Print and shaded views of the part. All mm, measured from the part's lowest x, y and z. A direction names the side the tool comes from. Give positions to 0.01 mm unless a question says otherwise; leave off trailing zeros. Loops run counter-clockwise (first coordinate to the right, second up) from the corner with the lowest first, then second, coordinate; pieces in that order, holes last. Notation, with made-up numbers: (31, -12.75) -> (47, -12.75) arc R20 cw to (47, 13.25) -> close; hole circle Ø4 at (-38.5, -18.75). An arc over 180 degrees is marked (long way). Answer as a JSON object with one key per item and string values. Group by question number.
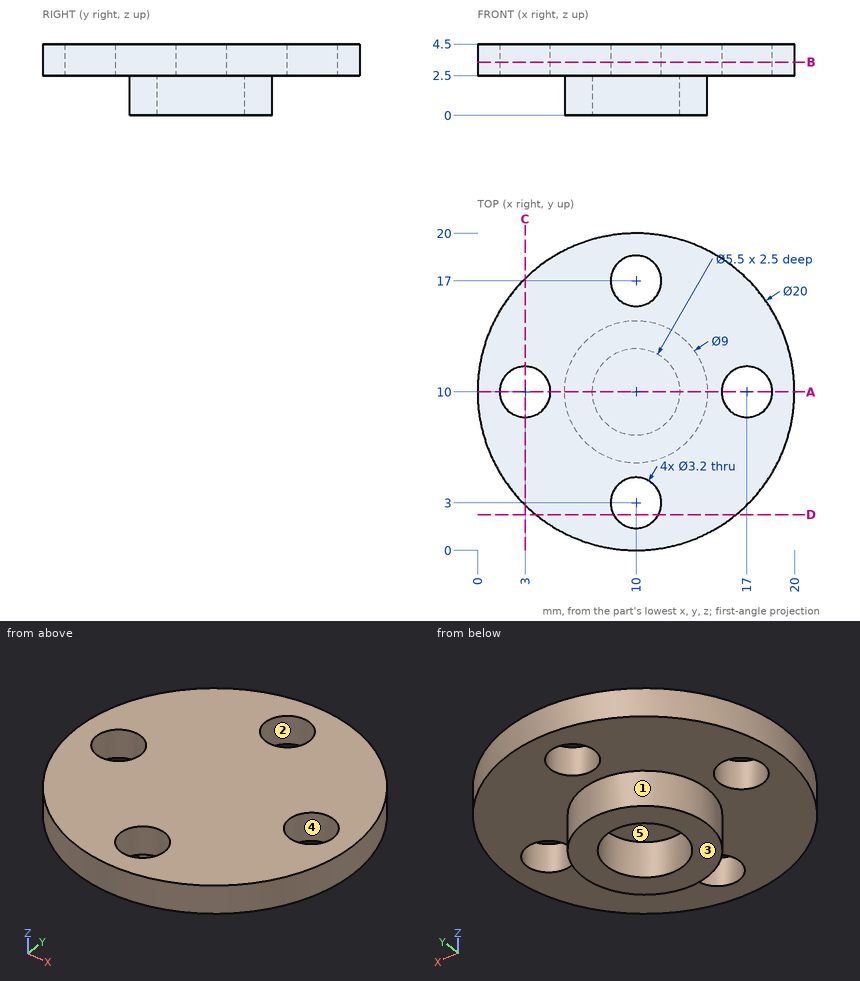
(1) Saw through at C-C on x = 3. List the corners of the cut face in (y, z), plus the area to 3 significant figures.
(2) 3-axis set-ups, long thin cutter, end or side, ignore diameter. For the marked faces 4 and 5: which of +Z, -Z, +X, -X, +Y, -Y reach the whole face in a straight line?
(3) Saw through at B-B on z = 3.35. List the corners of the cut face in (x, y), plus the area to 3 significant figures.
(4) Saw through at D-D on y = 2.25. List the corners of the cut face in (x, z).
(5) Pull direction X, two halves, no side cores. Call the marked faces 1, 2 and 3: pulls with the +X half, pulls with the -X half, needs draft (parallel to the pull), parting line crosses it, or undercut.
(6) Probe line 1 along Y through (x, z) = (10, 3.35); line 2 along Y through (x, z) = (11, 2.95); line 3 along Z through (x, y) = (15, 8). List the from-to ranges inside material, lowest first. Write a range as [from, to].
(7) Pin check, flat tips, straight feed: pin 1 (3 mm diameter, centred on x = 8, y = 3.5, fed in from -Z); pin 2 (1.5 mm diameter, centred on x = 11.5, z = 1, fed in from +Y); pin 3 (1 mm diameter, centred on x = 4, z = 4, fed in from +Y). Stop position of each tip, or through.
(8) Saw through at A-A on y = 10. List the corners of the cut face in (x, z), plus the area to 4 significant figures.
Calculated:
{
 "1": {"outline": "(2.86, 2.5) -> (8.4, 2.5) -> (8.4, 4.5) -> (2.86, 4.5) -> close; (11.6, 2.5) -> (17.14, 2.5) -> (17.14, 4.5) -> (11.6, 4.5) -> close", "area": "22.2 mm^2"},
 "2": {"face 4": "+Z, -Z", "face 5": "-Z"},
 "3": {"outline": "circle Ø20 at (10, 10); hole circle Ø3.2 at (3, 10); hole circle Ø3.2 at (10, 3); hole circle Ø3.2 at (10, 17); hole circle Ø3.2 at (17, 10)", "area": "282 mm^2"},
 "4": {"outline": "(3.68, 2.5) -> (8.59, 2.5) -> (8.59, 4.5) -> (3.68, 4.5) -> close; (11.41, 2.5) -> (16.32, 2.5) -> (16.32, 4.5) -> (11.41, 4.5) -> close"},
 "5": {"face 1": "parting line crosses it", "face 2": "undercut", "face 3": "needs draft"},
 "6": {"line 1": "y = [0, 1.4], [4.6, 15.4], [18.6, 20]", "line 2": "y = [0.05, 1.75], [4.25, 15.75], [18.25, 19.95]", "line 3": "z = [2.5, 4.5]"},
 "7": {"pin 1": "stops at z = 2.5", "pin 2": "stops at y = 14.44", "pin 3": "stops at y = 18.35"},
 "8": {"outline": "(0, 2.5) -> (1.4, 2.5) -> (1.4, 4.5) -> (0, 4.5) -> close; (4.6, 2.5) -> (5.5, 2.5) -> (5.5, 0) -> (7.25, 0) -> (7.25, 2.5) -> (12.75, 2.5) -> (12.75, 0) -> (14.5, 0) -> (14.5, 2.5) -> (15.4, 2.5) -> (15.4, 4.5) -> (4.6, 4.5) -> close; (18.6, 2.5) -> (20, 2.5) -> (20, 4.5) -> (18.6, 4.5) -> close", "area": "35.95 mm^2"}
}
